Geometry: see drawing. Coordinates: mm, zero at the bounding-box minimum. Round coordinates to 2 decimals unless told otherwise and drop trailing zeros. Loops run counter-clockwise (first coordinate to the right, second up) from the corner with the lowest first, then second, coordinate; pieces in that order, holes last. Notation, with made-up numbers: M 28,83.25 L 45,83.25 A22 ccw 45,109.25 Z; hole C 66,50.5 d9. An arc over 180 degrees is marked long. Answer as a JSON object with one key per item and string values.
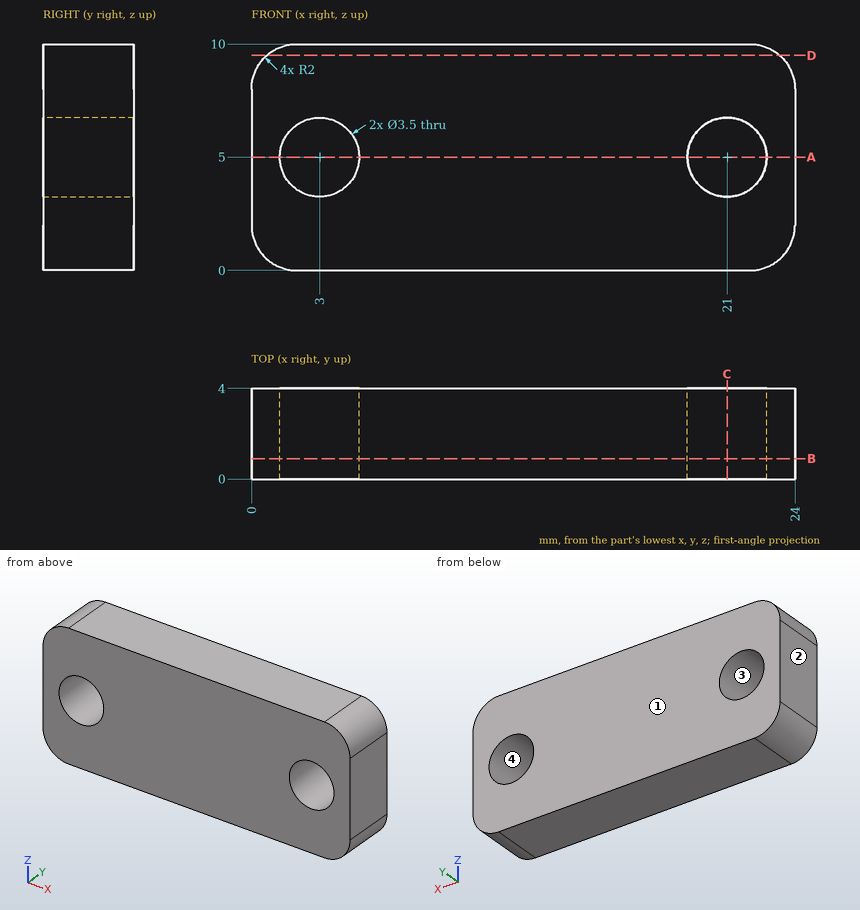
1) Pull-direction query (X, two-part tool) for the marked faces 1, 2, 3 and 4; classes: +X half, -X half, draft (parallel to the pull), parting line (faces both ways), or undercut.
Results:
{"face 1": "draft", "face 2": "-X half", "face 3": "undercut", "face 4": "undercut"}
2) Section query C-C (x = 21). Return the cut outline in (y, z), and give its area (3 significant figures).
Results:
{"outline": "M 0,0 L 4,0 L 4,3.25 L 0,3.25 Z; M 0,6.75 L 4,6.75 L 4,10 L 0,10 Z", "area": "26.0 mm2"}
3) Section query D-D (z = 9.5). Return the cut outline in (x, y), and give its area (3 significant figures).
Results:
{"outline": "M 0.68,0 L 23.32,0 L 23.32,4 L 0.68,4 Z", "area": "90.6 mm2"}
4) Section query A-A (z = 5). Return the cut outline in (x, y), and give its area (3 significant figures).
Results:
{"outline": "M 0,0 L 1.25,0 L 1.25,4 L 0,4 Z; M 4.75,0 L 19.25,0 L 19.25,4 L 4.75,4 Z; M 22.75,0 L 24,0 L 24,4 L 22.75,4 Z", "area": "68.0 mm2"}
5) Section query B-B (y = 0.9). Return the cut outline in (x, z), and give its area (3 significant figures).
Results:
{"outline": "M 0,2 A2 ccw 2,0 L 22,0 A2 ccw 24,2 L 24,8 A2 ccw 22,10 L 2,10 A2 ccw 0,8 Z; hole C 3,5 d3.5; hole C 21,5 d3.5", "area": "217 mm2"}
6) Ray query, line 1 (X direction, y = 2.85, z = 5); line 2 (Z direction, x = 21, y = 1.5); line 3 (X direction, y = 3.35, z = 6). Return the intervals inside material, ascending.
Results:
{"line 1": "0 to 1.25, 4.75 to 19.25, 22.75 to 24", "line 2": "0 to 3.25, 6.75 to 10", "line 3": "0 to 1.56, 4.44 to 19.56, 22.44 to 24"}
